```python
from build123d import *

# Parameters (mm, degrees)
BOSS_EXTRUDE1_DEPTH            = 12.5
CUT_EXTRUDE1_REACH             = 42.954
CUT_EXTRUDE1_DIRECTION_2_REACH = 42.954
FILLET1_R                      = 2
BOSS_EXTRUDE2_DEPTH            = 24
BOSS_EXTRUDE2_DEPTH_BACK       = 24
SKETCH3_R                      = 4.5


with BuildPart() as part:
    # Sketch1 → Boss-Extrude1 (new body)
    with BuildSketch(Plane(origin=(0, 0, 0), x_dir=(1, 0, 0), z_dir=(0, 1, 0))):
        with BuildLine():
            Line((13.35, -10), (15, -10))
            Line((15, -10), (15, 10))
            Line((15, 10), (-15, 10))
            Line((-15, 10), (-15, -10))
            Line((-15, -10), (-13.35, -10))
            ThreePointArc((-13.35, -10), (-11.935786438, -10.585786438), (-11.35, -12))
            Line((-11.35, -12), (-11.35, -36))
            Line((-11.35, -36), (11.35, -36))
            Line((11.35, -36), (11.35, -12))
            ThreePointArc((11.35, -12), (11.935786438, -10.585786438), (13.35, -10))
        make_face()
    extrude(amount=BOSS_EXTRUDE1_DEPTH)

    # Cut-Extrude1: up to this face of the body (flat: up to its plane)
    cut_extrude1_end = Plane(part.part.faces().sort_by_distance((-11.35, 6.25, 24))[0])
    # Sketch2 → Cut-Extrude1 (cut, up to the picked face)
    with BuildSketch(Plane(origin=(0, 0, 0), x_dir=(0, 0, -1), z_dir=(1, 0, 0)), mode=Mode.PRIVATE) as cut_extrude1_sk1:
        Polygon((-36, 0), (-32.5, 12.5), (-36, 12.5), align=None)
    cut_extrude1_tool1 = split(extrude(cut_extrude1_sk1.sketch, amount=-CUT_EXTRUDE1_REACH, mode=Mode.PRIVATE), bisect_by=cut_extrude1_end, keep=Keep.BOTH, mode=Mode.PRIVATE)
    add(cut_extrude1_tool1.solids().sort_by(Axis((0, 8.333333, 34.833333), (-1, 0, 0)))[0], mode=Mode.SUBTRACT)

    # Cut-Extrude1 direction 2: up to this face of the body (flat: up to its plane)
    cut_extrude1_direction_2_end = Plane(part.part.faces().sort_by_distance((11.35, 6.25, 24))[0])
    # Sketch2 → Cut-Extrude1 direction 2 (cut, up to the picked face)
    with BuildSketch(Plane(origin=(0, 0, 0), x_dir=(0, 0, -1), z_dir=(1, 0, 0)), mode=Mode.PRIVATE) as cut_extrude1_direction_2_sk1:
        Polygon((-36, 0), (-32.5, 12.5), (-36, 12.5), align=None)
    cut_extrude1_direction_2_tool1 = split(extrude(cut_extrude1_direction_2_sk1.sketch, amount=CUT_EXTRUDE1_DIRECTION_2_REACH, mode=Mode.PRIVATE), bisect_by=cut_extrude1_direction_2_end, keep=Keep.BOTH, mode=Mode.PRIVATE)
    add(cut_extrude1_direction_2_tool1.solids().sort_by(Axis((0, 8.333333, 34.833333), (1, 0, 0)))[0], mode=Mode.SUBTRACT)

    # Fillet1
    fillet1_edges = [part.edges().sort_by_distance(p)[0] for p in [
        (0, 12.5, 32.5),
        (11.35, 6.25, 34.25),
        (-11.35, 6.25, 34.25),
    ]]
    fillet(fillet1_edges, radius=FILLET1_R)

    # Sketch3 → Boss-Extrude2 (add, two sides: drawn at the far end of the back side and taken through both)
    with BuildSketch(Plane(origin=(0, 0, 0), x_dir=(0, 0, -1), z_dir=(1, 0, 0)).offset(-BOSS_EXTRUDE2_DEPTH_BACK)):
        with Locations((0, 6.25)):
            Circle(SKETCH3_R)
    extrude(amount=BOSS_EXTRUDE2_DEPTH + BOSS_EXTRUDE2_DEPTH_BACK)


solid = part.part
```
For this review, take the finished solid that the model builds, in its own axes (mm). A direction names the side the tool comes from. Round coordinates to 2 decimals unless told otherwise and drop trailing zeros. Write each loop counter-clockwise with the first axis right and the second up, starting at its lowest first coordinate (ties: lowest second). Pieces come first, ordered by that corner, then holes. Notation, with made-up numbers: M -26.5,-2 L -3.5,-2 A33 cw -3.5,34 Z; hole C 2,-39.75 d2. An arc over 180 degrees is marked long. One line per item, written item: value. Start each with the question number.
(1) We need section B-B (z = 0). Give the boundary of the cut face in (x, y).
(2) We need section C-C (z = -6). Give the boundary of the cut face in (x, y).
(3) Machinability: for faces 1 (the flat face through (11.35, 6, 23)), 2 (the flat face through (-15, 6, -5)), 3 (the cylindrical face through (10.75, 6.46, 33.6)), 4 (the flat face through (-14, 6, 10)), 5 (the cylindrical face through (19.44, 3.51, 3.57)), which of the approach directions +Z, -Z, +X, -X, +Y, -Y give a long, thin tool a straight path to every point of the face, cutting with its end or side? Answer none if there is none.
(4) Insertion check: pin 1 (1.8 mm diameter, centred on x = -14.5, y = 7.5, fed in from +Z); pin 2 (1 mm diameter, centred on y = 5.5, z = 21.5, fed in from -X); pin 3 (4 mm diameter, centred on y = 3, z = 27, fed in from +X); pin 4 (6 mm diameter, centred on y = 3.5, z = -4.5, fed in from -X). Each pin has a flat end and moves straight along its axis. Give the tip position at first contact, or say it passes through.
(5) We need section D-D (x = 10). Give the boundary of the cut face in (y, z).
(6) Wall thickness on line 1 (X direction, y = 4, z = 33); line 2 (X direction, y = 7, z = 21); line 3 (Z direction, x = -17, y = 6.25): over which ranges is each line inside the solid? List them lowest first.
(7) We need section A-A (x = -0.5). Give the boundary of the cut face in (y, z), and give its area (3 significant figures).
Result:
1. outline: M -24,1.75 L -15,1.75 L -15,0 L 15,0 L 15,1.75 L 24,1.75 L 24,10.75 L 15,10.75 L 15,12.5 L -15,12.5 L -15,10.75 L -24,10.75 Z
2. outline: M -15,0 L 15,0 L 15,12.5 L -15,12.5 Z
3. face 1: +Z, +X, +Y, -Y
3. face 2: -X
3. face 3: +Z, +X, +Y
3. face 4: +Z, -X, +Y, -Y
3. face 5: +X
4. pin 1: z = 10
4. pin 2: x = -11.35
4. pin 3: x = 11.35
4. pin 4: x = -24
5. outline: M 0,-10 L 12.5,-10 L 12.5,30.98 A2 ccw 11.64,32.63 L 0,35.89 Z
6. line 1: -11.34 to 11.34
6. line 2: -11.35 to 11.35
6. line 3: -4.5 to 4.5
7. outline: M 0,-10 L 12.5,-10 L 12.5,30.98 A2 ccw 11.04,32.91 L 0,36 Z
7. area: 553 mm²
